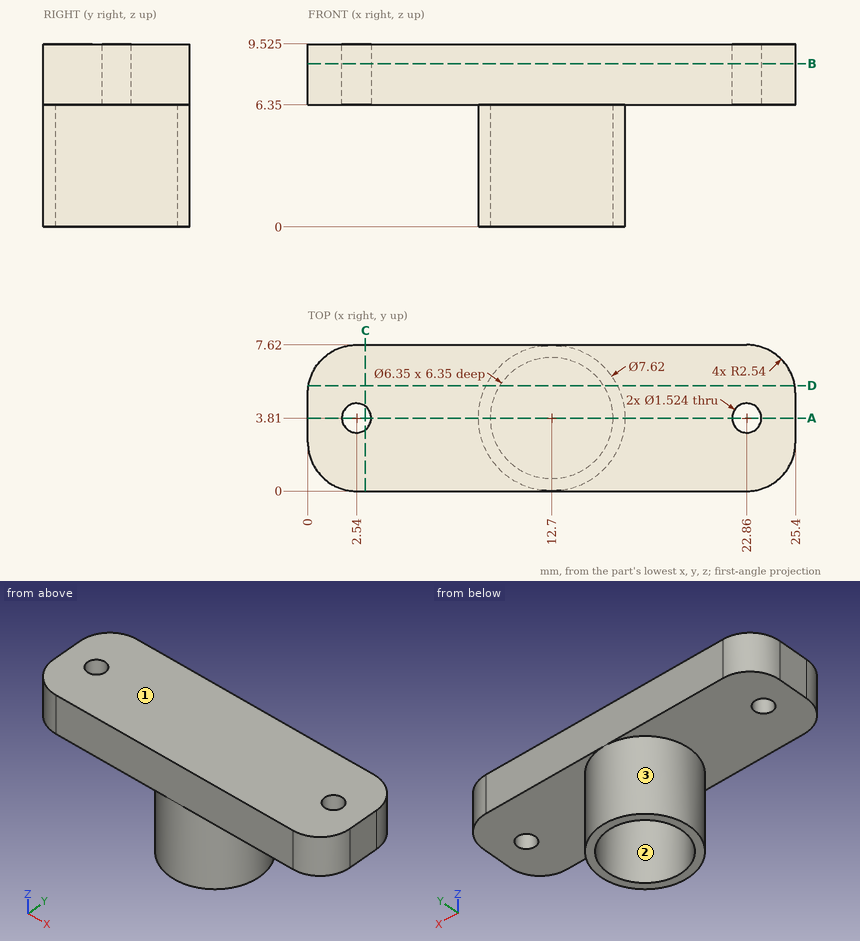
Design review of the part shown in the three views and the two pictorial views. Dimensions are in mm from the part's minimum x, y and z. Round coordinates to 2 decimals unless told otherwise and drop trailing zeros. Write each loop counter-clockwise with the first axis right and the second up, starting at its lowest first coordinate (ties: lowest second). Pieces come first, ordered by that corner, then holes. Notation, with made-up numbers: (48, 77) - (65, 77) arc R22 ccw to (65, 103) - close; hole circle Ø3 at (9.25, 34). An arc over 180 degrees is marked (long way). Return JSON: item names as keys, results as strings. Group by question number.
Item 1: We need section C-C on x = 3. Write out the cut boundary in (y, z) (3 decimals).
Item 2: The part is to be moulded in two halves that separate along X. For the marked faces 1, 2 and 3, say which applies: pulls with the +X half, pulls with the -X half, needs draft (parallel to the pull), parting line crosses it, or undercut.
Item 3: For probe 1 along Y at (x, z) = (12.7, 4) (3 decimals); probe 2 along Z at (x, y) = (23, 0.5) (3 decimals); probe 3 along Y at (x, z) = (2.54, 8.25), list the stretches that pass through material, from the lowest coordinate up. Write a range as [from, to].
Item 4: We need section B-B on z = 8.5. Write out the cut boundary in (x, y), and give its area (3 significant figures).
Item 5: Insertion check: P1, Ø3, axis at x = 13, y = 4, coming from the -Z side. The pin has a flat end and moves straight along its axis. Give the tip position at first contact, or say it passes through.
Item 6: We need section D-D on y = 5.5. Write out the cut boundary in (x, z) (3 decimals), and give its area (3 significant figures).
Item 7: We need section A-A on y = 3.81. Write out the cut boundary in (x, z) (3 decimals), and give its area (3 significant figures).
Model answer:
{
 "1": {"outline": "(0, 6.35) - (3.203, 6.35) - (3.203, 9.525) - (0, 9.525) - close; (4.417, 6.35) - (7.62, 6.35) - (7.62, 9.525) - (4.417, 9.525) - close"},
 "2": {"face 1": "needs draft", "face 2": "undercut", "face 3": "parting line crosses it"},
 "3": {"probe 1": "y = [0, 0.635], [6.985, 7.62]", "probe 2": "z = [6.35, 9.525]", "probe 3": "y = [0, 3.05], [4.57, 7.62]"},
 "4": {"outline": "(0, 2.54) arc R2.54 ccw to (2.54, 0) - (22.86, 0) arc R2.54 ccw to (25.4, 2.54) - (25.4, 5.08) arc R2.54 ccw to (22.86, 7.62) - (2.54, 7.62) arc R2.54 ccw to (0, 5.08) - close; hole circle Ø1.52 at (2.54, 3.81); hole circle Ø1.52 at (22.86, 3.81)", "area": "184 mm²"},
 "5": {"P1": "stops at z = 6.35"},
 "6": {"outline": "(0.035, 6.35) - (9.285, 6.35) - (9.285, 0) - (10.012, 0) - (10.012, 6.35) - (15.388, 6.35) - (15.388, 0) - (16.115, 0) - (16.115, 6.35) - (25.365, 6.35) - (25.365, 9.525) - (0.035, 9.525) - close", "area": "89.7 mm²"},
 "7": {"outline": "(0, 6.35) - (1.778, 6.35) - (1.778, 9.525) - (0, 9.525) - close; (3.302, 6.35) - (8.89, 6.35) - (8.89, 0) - (9.525, 0) - (9.525, 6.35) - (15.875, 6.35) - (15.875, 0) - (16.51, 0) - (16.51, 6.35) - (22.098, 6.35) - (22.098, 9.525) - (3.302, 9.525) - close; (23.622, 6.35) - (25.4, 6.35) - (25.4, 9.525) - (23.622, 9.525) - close", "area": "79.0 mm²"}
}
